Build history of the part. All positions in model axes, mm. Give positions to 0.01 mm unless a question says otherwise; leave off trailing zeros. Write each loop counter-clockwise with the first axis right and the second up, starting at its lowest first coordinate (ties: lowest second). Pieces come first, ordered by that corner, then holes. Notation, with made-up numbers: (5, 62.25) - (49, 62.25) arc R17 ccw to (49, 81.25) - close; hole circle Ø6 at (-28.75, 77.5). An arc over 180 degrees is marked (long way). Use one line per item in the form item = value. Start each with the question number.
from build123d import *

# Parameters (mm, degrees)
SKETCH1_R                       = 1.175
PRINTED_NUT_AF5P4_H2P4_DEPTH    = 2.4
ACTUAL_MATCHING_FEMALE_P1_PITCH = 1


with BuildPart() as part:
    # Sketch1 → Printed_nut_AF5p4_H2p4 (new body)
    with BuildSketch(Plane.XY):
        Polygon((3.117691454, 0), (1.558845727, 2.7), (-1.558845727, 2.7), (-3.117691454, 0), (-1.558845727, -2.7), (1.558845727, -2.7), align=None)
        Circle(SKETCH1_R, mode=Mode.SUBTRACT)
    extrude(amount=PRINTED_NUT_AF5P4_H2P4_DEPTH)

    # Actual_matching_female_P1: the profile of 3DSketch1 screwed along a right-hand helix of 3 turns, 8 arcs to a turn; built about Z, then put on its axis
    actual_matching_female_p1_z = Axis((0, 0, 0), (0, 0, 1))
    actual_matching_female_p1_corners = [(1.075, 0, -0.52), (1.65, 0, -0.22), (1.65, 0, 0.22), (1.075, 0, 0.52)]
    with BuildLine(mode=Mode.PRIVATE) as actual_matching_female_p1_profile:
        Line(actual_matching_female_p1_corners[0], actual_matching_female_p1_corners[1])
        Line(actual_matching_female_p1_corners[1], actual_matching_female_p1_corners[2])
        Line(actual_matching_female_p1_corners[2], actual_matching_female_p1_corners[3])
        Line(actual_matching_female_p1_corners[3], actual_matching_female_p1_corners[0])
    actual_matching_female_p1_cap = Face(actual_matching_female_p1_profile.wire())
    actual_matching_female_p1_turn_angles = [0, 22.5, 45, 67.5, 90, 112.5, 135, 157.5, 180, 202.5, 225, 247.5, 270, 292.5, 315, 337.5, 360]
    actual_matching_female_p1_turn_weights = [1, 0.9238795325112867, 1, 0.9238795325112867, 1, 0.9238795325112867, 1, 0.9238795325112867, 1, 0.9238795325112867, 1, 0.9238795325112867, 1, 0.9238795325112867, 1, 0.9238795325112867, 1]
    actual_matching_female_p1_turn_rails = [Edge.make_bspline([Vector(p[0], p[1], 0).rotate(actual_matching_female_p1_z, actual_matching_female_p1_turn_angles[k]) / actual_matching_female_p1_turn_weights[k] + Vector(0, 0, p[2] + ACTUAL_MATCHING_FEMALE_P1_PITCH * actual_matching_female_p1_turn_angles[k] / 360) for k in range(17)], [0, 0, 0, 1, 1, 2, 2, 3, 3, 4, 4, 5, 5, 6, 6, 7, 7, 8, 8, 8], 2, actual_matching_female_p1_turn_weights) for p in actual_matching_female_p1_corners]
    actual_matching_female_p1_turn_sides = [Face.make_surface_from_curves(actual_matching_female_p1_turn_rails[p[0]], actual_matching_female_p1_turn_rails[p[1]]) for p in [(0, 1), (1, 2), (2, 3), (3, 0)]]
    actual_matching_female_p1 = Plane(origin=(0, 0, 0.25005), x_dir=(1, 0, 0), z_dir=(0, 0, 1)) * Solid(Shell([*[p.moved(Location((0, 0, ACTUAL_MATCHING_FEMALE_P1_PITCH * i))) for i in range(3) for p in actual_matching_female_p1_turn_sides], actual_matching_female_p1_cap, actual_matching_female_p1_cap.rotate(actual_matching_female_p1_z, 1080).moved(Location((0, 0, ACTUAL_MATCHING_FEMALE_P1_PITCH * 1080 / 360)))]))
    add(actual_matching_female_p1, mode=Mode.SUBTRACT)


solid = part.part
(1) Wall check: line 1 (Z direction, x = -1.5, y = 0.15); line 2 (Z direction, x = -1.25, y = 0.45); line 3 (Z direction, x = 1.25, y = 0.6). Give the ranges that are in metal, low to high. Write a range as from..to.
(2) Pin check, flat tips, straight feed: pin 1 Ø2.5 at (x, y) = (0, 0) entering from -Z; pin 2 Ø1 at (y, z) = (1.5, 1.5) entering from +X; pin 3 Ø2 at (x, y) = (0, 0) entering from -Z. Stop position of each tip, or through.
(3) Cut at B-B, the plane y = -2.2. Give the cut face in (x, z), then the cut area to 3 significant figures.
(4) Cut at A-A, the plane y = -1.55. State how many separate pieces and enclosed holes the cut face has, then the cut area to 3 significant figures.
Solution:
q1.line_1 = 0..0.44, 1.03..1.44, 2.03..2.4
q1.line_2 = 0..0.31, 1.08..1.31, 2.08..2.31
q1.line_3 = 0.68..0.96, 1.68..1.96
q2.pin_1 = 0
q2.pin_2 = 2.54
q2.pin_3 = through
q3.outline = (-1.85, 0) - (1.85, 0) - (1.85, 2.4) - (-1.85, 2.4) - close
q3.area = 8.87 mm2
q4.separate_pieces = 1
q4.enclosed_holes = 2
q4.area = 9.52 mm2
